Read the model definition and answer for the solid it produces. Units are mm, in the model's axes. Face numbers are marked on the shaded views. A direction names the side the tool comes from. Coordinates: 2 decimals unless noted, no trailing zeros. Order: outer loops, then holes, each group sorted by start corner. A loop starts at its lowest first (then second) coordinate and runs counter-clockwise, first axis right, second up. Notation, with made-up numbers: (-38, -29.75) -> (-29, -29.75) arc R30 cw to (-29, 1.25) -> close; hole circle Ø4 at (16, 81.25). An arc over 180 degrees is marked (long way). Answer as a JSON object with one key per item and string values. Group by question number.
1) A tool of negligible diameter and unlimited length cuts with its end or side. For the marked faces 5 and 6, from which of +Z, -Z, +X, -X, +Y, -Y can it reach the whole face along a straight path? Write none if from no direction.
2) Section C-C on y = -29 is taken. Determine the outline of the cut face in (x, z).
3) Determine the mould class of the marked faces 1, 2, 3 and 4 for opening direction Z: released by +Z, released by -Z, zero draft, split by the parting line, or undercut.
4) Consider L1, parallel to Z at x = 31, y = 0; L2, parallel to Z at x = 42, y = 0; L3, parallel to Y at x = 28.75, z = 15. Determine where each line is inside the solid, lowest interval first.
5) Section B-B on x = 10 is taken. Determine the outline of the cut face in (y, z).
6) Section A-A on z = 15 is taken. Count the separate pieces of the cut face and the enclosed holes in it, and give its area (3 significant figures).
7) Given pin 1 (18 mm diameter, centred on x = 10, z = 15, fed in from -Y); pin 2 (8 mm diameter, centred on x = -14, y = 12, fed in from +Z); pin 3 (8 mm diameter, centred on y = -15.5, z = 53.5, fed in from +X); pin 4 (10 mm diameter, centred on y = 1, z = 11.5, fed in from +X), each flat-ended and moving along its own axis, determine where each tip first touches the part or whether it passes through.
from build123d import *

# Parameters (mm, degrees)
F0_W           = 90
F0_H           = 70
F1_DEPTH       = 30
F2_R           = 34.99999
F3_R           = 10
F4_DEPTH       = 70.001
F6_D           = 10
F6_DEPTH       = 35
F6_CBORE_D     = 20
F6_CBORE_DEPTH = 10
F6_TIP         = 3.0043030951
F7_R           = 15
F8_DEPTH       = 30


# Not quite as in the source:
# - a fillet or chamfer is up to 0.001 mm smaller than in the source, because OpenCascade refuses the exact size


with BuildPart() as f1:
    # F0 (on Top) → F1 (new body)
    with BuildSketch(Plane.XY):
        Rectangle(F0_W, F0_H)
    extrude(amount=F1_DEPTH)

    # F2 (radius 35 in the source; OpenCascade refuses exactly that, so slightly less here)
    f2_edges = [f1.edges().sort_by_distance(p)[0] for p in [
        (-45, 35, 15),
        (-45, -35, 15),
    ]]
    fillet(f2_edges, radius=F2_R)

    # F3 (on face) → F4 (cut, through all)
    with BuildSketch(Plane.XZ.offset(35)):
        with Locations((10, 15)):
            Circle(F3_R)
    extrude(amount=-F4_DEPTH, mode=Mode.SUBTRACT)

    # F6
    with Locations(Plane.YZ.offset(45)):
        with Locations((0, 15)):
            CounterBoreHole(F6_D / 2, F6_CBORE_D / 2, F6_CBORE_DEPTH, depth=F6_DEPTH)
            with Locations((0, 0, -(F6_DEPTH + F6_TIP / 2))):  # 118° drill point
                Cone(0, F6_D / 2, F6_TIP, mode=Mode.SUBTRACT)

    # F7 (on face) → F8 (join)
    with BuildSketch(Plane.XY.offset(30)):
        with Locations((10, 0)):
            Circle(F7_R)
    extrude(amount=F8_DEPTH)


solid = f1.part
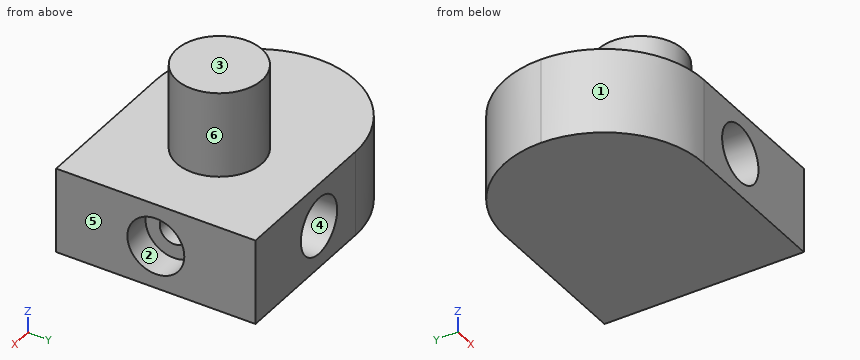
Worked answers:
{
 "1": {"face 5": "+Z, -Z, +X, +Y, -Y", "face 6": "+Z"},
 "2": {"outline": "(-29.6, 0) -> (45, 0) -> (45, 30) -> (-29.6, 30) -> close; hole circle Ø20 at (10, 15)"},
 "3": {"face 1": "zero draft", "face 2": "undercut", "face 3": "released by +Z", "face 4": "undercut"},
 "4": {"L1": "z = 0 to 10, 20 to 30", "L2": "z = 0 to 5, 25 to 30", "L3": "y = -35 to -5, 5 to 35"},
 "5": {"outline": "(-35, 0) -> (35, 0) -> (35, 5) -> (-35, 5) -> close; (-35, 25) -> (35, 25) -> (35, 30) -> (15, 30) -> (15, 60) -> (-15, 60) -> (-15, 30) -> (-35, 30) -> close"},
 "6": {"separate pieces": "3", "enclosed holes": "0", "area": "4,020 mm²"},
 "7": {"pin 1": "passes through", "pin 2": "stops at z = 30", "pin 3": "stops at x = 19.63", "pin 4": "stops at x = 35"}
}
